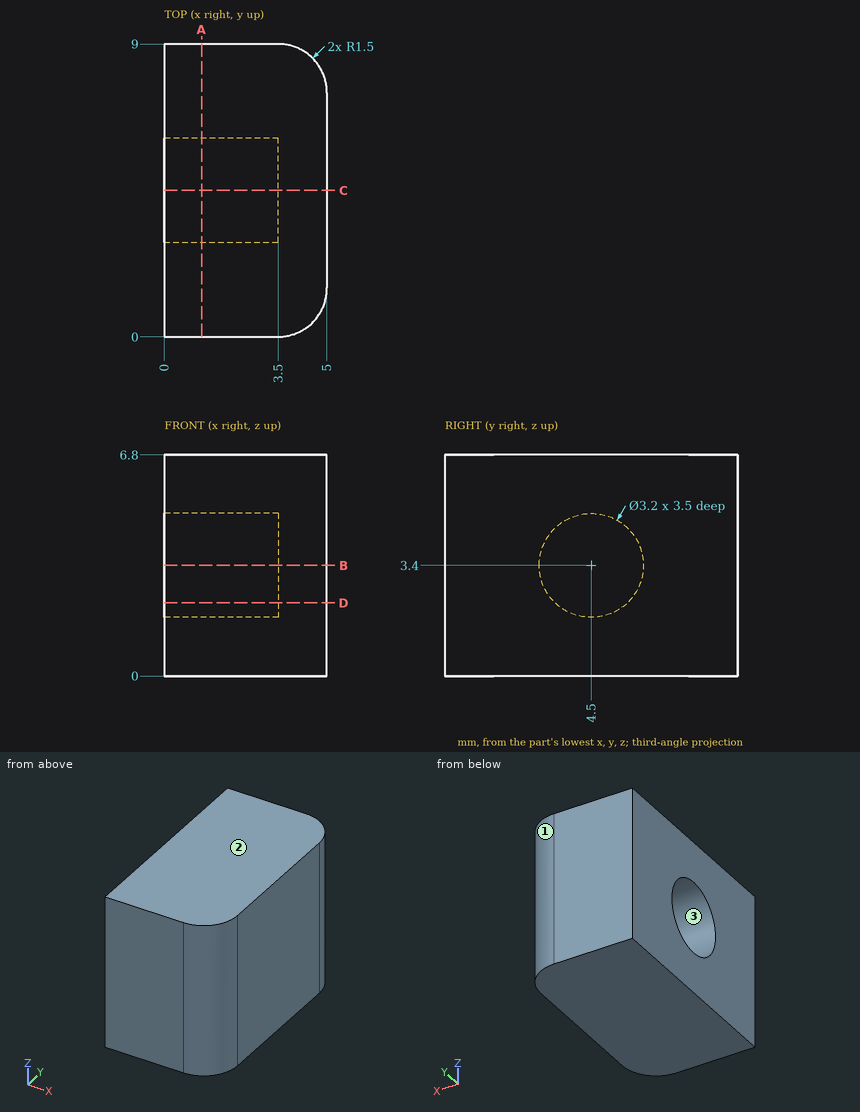
Job drawing, mm, ordinate dimensions from the low corner. One solid piece. Round coordinates to 2 decimals unless told otherwise and drop trailing zeros. Loops run counter-clockwise (first coordinate to the right, second up) from the corner with the lowest first, then second, coordinate; pieces in that order, holes last. Notation, with made-up numbers: (2, 57) -> (15, 57) arc R7 cw to (15, 65) -> close; hole circle Ø6 at (22, 1). An arc over 180 degrees is marked (long way). Use a Markdown table: item, result.
1) Pull direction Y, two halves, no side cores. Call the marked faces 1, 2 and 3: pulls with the +Y half, pulls with the -Y half, needs draft (parallel to the pull), parting line crosses it, or undercut.
The answers:
| item | result |
|---|---|
| face 1 | pulls with the +Y half |
| face 2 | needs draft |
| face 3 | undercut |
2) Drop a flat-ended pin along its axis: pin 1 Ø1 at (y, z) = (4.5, 4) entering from -X. Give the stop position or say it passes through.
The answers:
| item | result |
|---|---|
| pin 1 | stops at x = 3.5 |
3) Cut at C-C, the plane y = 4.5. List the corners of the cut face in (x, z), and give its area (3 significant figures).
The answers:
| item | result |
|---|---|
| outline | (0, 0) -> (5, 0) -> (5, 6.8) -> (0, 6.8) -> (0, 5) -> (3.5, 5) -> (3.5, 1.8) -> (0, 1.8) -> close |
| area | 22.8 mm2 |
4) Cut at D-D, the plane z = 2.25. List the corners of the cut face in (x, y), and give its area (3 significant figures).
The answers:
| item | result |
|---|---|
| outline | (0, 0) -> (3.5, 0) arc R1.5 ccw to (5, 1.5) -> (5, 7.5) arc R1.5 ccw to (3.5, 9) -> (0, 9) -> (0, 5.61) -> (3.5, 5.61) -> (3.5, 3.39) -> (0, 3.39) -> close |
| area | 36.2 mm2 |
5) Cut at A-A, the plane x = 1.15. List the corners of the cut face in (y, z).
The answers:
| item | result |
|---|---|
| outline | (0, 0) -> (9, 0) -> (9, 6.8) -> (0, 6.8) -> close; hole circle Ø3.2 at (4.5, 3.4) |
6) Cut at B-B, the plane z = 3.4. List the corners of the cut face in (x, y), and give its area (3 significant figures).
The answers:
| item | result |
|---|---|
| outline | (0, 0) -> (3.5, 0) arc R1.5 ccw to (5, 1.5) -> (5, 7.5) arc R1.5 ccw to (3.5, 9) -> (0, 9) -> (0, 6.1) -> (3.5, 6.1) -> (3.5, 2.9) -> (0, 2.9) -> close |
| area | 32.8 mm2 |
7) Probe line 1 (Z direction, x = 1.3, y = 4.5); line 2 (Y direction, x = 1.9, z = 3.5); line 3 (Y direction, x = 2.7, z = 4.5). List the from-to ranges inside material, lowest first. Write a range as [from, to].
The answers:
| item | result |
|---|---|
| line 1 | z = [0, 1.8], [5, 6.8] |
| line 2 | y = [0, 2.9], [6.1, 9] |
| line 3 | y = [0, 3.34], [5.66, 9] |
